Geometry check sheet. Reference: the model listing, model coordinates, mm. Give positions to 0.01 mm unless a question says otherwise; leave off trailing zeros. Loops run counter-clockwise (first coordinate to the right, second up) from the corner with the lowest first, then second, coordinate; pieces in that order, holes last. Notation, with made-up numbers: (10, 80) -> (15, 80) arc R16 ccw to (15, 94) -> close; hole circle Ø7 at (-15.75, 33.25). An arc over 180 degrees is marked (long way). One line per item, written item: value. Start each with the question number.
(1) Sectioned sample at B-B, the plane z = -124. Record the cut outline in (x, y), then the cut area to 3 significant figures.
(2) Draft check along Z on faces 1 (the face through (15.83, 103.48, -178.32)), 2 (the face through (15.83, 11.61, -171.28)), 3 (the face through (15.8, 89.7, -146.8)), 4 (the face through (15.83, 34.47, -118.71)). Enter one of: pulls with the +Z half, pulls with the -Z half, needs draft (parallel to the pull), parting line crosses it, or undercut.
(3) Sectioned sample at A-A, the plane y = 65.5. Record the cut outline in (x, z), then the cut area to 3 significant figures.
(4) Scan lines: line 1 along Z through (x, y) = (14.5, 36.5); line 2 along Z through (x, y) = (16.25, 58.5); line 3 along Y through (x, z) = (15, -130). Record each from-to range of solid material in increasing order. Write a range as from..to.
(5) Sectioned sample at C-C, the plane z = -134.5. Record the cut outline in (x, y).
(6) Sectioned sample at D-D, the plane x = 14.5. State how many separate pieces and enclosed holes the cut face has, then the cut area to 3 significant figures.
Autodesk Inventor part; units mm, degrees
ref_plane "Work Plane1" through (12.7, 0, 0) normal (1, 0, 0) x (0, 0, -1)
ref_plane "YZ Plane" through (0, 0, 0) normal (1, 0, 0) x (0, 1, 0)
ref_plane "XZ Plane" through (0, 0, 0) normal (0, 1, 0) x (-1, 0, 0)
sketch "Sketch1" plane through (0, 0, 0) normal (1, 0, 0) x (0, 1, 0)
  line L0 (111.125, 190.5) -> (68.3957, 190.5)
  line L1 (20.2274, 160.5064) -> (-11.1661, 102.5705)
  arc A0 (-11.1661, 102.5705) -> (-11.1661, 90.4695) centre (0, 96.52) ccw
  line L2 (-11.1661, 90.4695) -> (7.6076, 55.8231)
  arc A1 (-11.1661, 6.0505) -> (-11.1661, -6.0505) centre (0, 0) ccw
  line L3 (-11.1661, -6.0505) -> (7.6076, -40.6969)
  arc A2 (-11.1661, -90.4695) -> (-11.3095, -102.2979) centre (0, -96.52) ccw
  line L4 (-11.3095, -102.2979) -> (18.6694, -160.9782)
  line L5 (67.5494, -190.5) -> (111.125, -190.5)
  line L6 (111.125, -190.5) -> (111.125, 190.5)
  arc A3 (20.2274, 160.5064) -> (68.3957, 190.5) centre (42.5128, 178.392) ccw
  arc A4 (67.5494, -190.5) -> (18.6694, -160.9782) centre (42.5128, -176.727) ccw
  circle A5 centre (42.5128, 178.392) radius 4.7625 construction
  circle A6 centre (34.925, -92.075) radius 7.9375
  circle A7 centre (73.5908, -125.0234) radius 6.35 construction
  circle A8 centre (42.5128, -176.727) radius 4.7625 construction
  line L7 (111.125, 0) -> (0, 0) construction
  circle A9 centre (0, 96.52) radius 2.4892 construction
  circle A10 centre (0, 0) radius 2.4892 construction
  circle A11 centre (0, -96.52) radius 2.4892 construction
  line L8 (-11.1661, 6.0505) -> (7.6076, 40.6969)
  arc A12 (7.6076, 40.6969) -> (7.6076, 55.8231) centre (-6.35, 48.26) ccw
  line L9 (-11.1661, -90.4695) -> (7.6076, -55.8231)
  arc A13 (7.6076, -55.8231) -> (7.6076, -40.6969) centre (-6.35, -48.26) ccw
  line L10 (-6.35, -48.26) -> (-6.35, 48.26) construction
  line L11 (-6.35, 0) -> (0, 0) construction
  circle A14 centre (0, 96.52) radius 3.175
  circle A15 centre (0, 0) radius 3.175
  circle A16 centre (0, -96.52) radius 3.175
  circle A17 centre (46.0375, 122.682) radius 3.5687 construction
  circle A18 centre (20.6375, 122.682) radius 3.5687 construction
  circle A19 centre (46.0375, 122.682) radius 3.175
  circle A20 centre (20.6375, 122.682) radius 3.175
  line L12 (0, 96.52) -> (-12.7, 96.52) construction
  circle A21 centre (99.3625, 57.065) radius 2.0193
  circle A22 centre (47.625, -17.78) radius 2.0193
  circle A23 centre (99.3625, 31.665) radius 2.0193
  circle A24 centre (73.9625, 57.065) radius 2.0193
  circle A25 centre (73.9625, 31.665) radius 2.0193
  circle A26 centre (47.625, -43.18) radius 2.0193
  circle A27 centre (22.225, -17.78) radius 2.0193
  circle A28 centre (22.225, -43.18) radius 2.0193
  circle A29 centre (85.725, 107.103) radius 7.9375
  line L13 (-12.7, 173.6352) -> (-12.7, -210.2893) construction
  circle A30 centre (85.725, 107.103) radius 17.78 construction
  circle A31 centre (79.375, 147.2439) radius 22.86 construction
  circle A32 centre (42.5128, 178.392) radius 25.4 construction
  line L14 (110.475, 71.035) -> (60.975, 71.035) construction
  line L15 (60.975, 71.035) -> (60.975, -72.669) construction
  line L16 (60.975, -72.669) -> (110.475, -72.669) construction
  line L17 (110.475, -72.669) -> (110.475, 71.035) construction
  line L18 (58.7375, 86.554) -> (9.2375, 86.554) construction
  line L19 (9.2375, 86.554) -> (9.2375, -57.15) construction
  line L20 (9.2375, -57.15) -> (58.7375, -57.15) construction
  line L21 (58.7375, -57.15) -> (58.7375, 86.554) construction
  line L22 (9.525, 127) -> (-15.875, 127) construction
  line L23 (-15.875, 127) -> (-15.875, -177.8) construction
  line L24 (-15.875, -177.8) -> (9.525, -177.8) construction
  line L25 (9.525, -177.8) -> (9.525, 127) construction
  circle A33 centre (34.925, -92.075) radius 17.78 construction
  circle A34 centre (73.5908, -125.0234) radius 28.575 construction
  circle A35 centre (42.5128, -176.727) radius 31.75 construction
  circle A36 centre (102.0089, 180.2336) radius 2.413
  circle A37 centre (89.3089, 182.1987) radius 2.413
  circle A38 centre (102.0089, -180.2336) radius 2.413
  circle A39 centre (89.3089, -182.1987) radius 2.413
  circle A40 centre (79.375, 147.2439) radius 14.2875
  circle A41 centre (66.675, 254) radius 60.325 construction
  circle A42 centre (66.675, -254) radius 60.325 construction
  circle A43 centre (73.5908, -125.0234) radius 14.2875
  circle A44 centre (80.899, -155.6385) radius 47.527 construction
  circle A45 centre (100.0125, -85.369) radius 3.175
  circle A46 centre (74.6125, -85.369) radius 3.175
  circle A47 centre (100.0125, -85.369) radius 6.35 construction
  circle A48 centre (74.6125, -85.369) radius 6.35 construction
  circle A49 centre (46.0375, 122.682) radius 6.35 construction
  circle A50 centre (20.6375, 122.682) radius 6.35 construction
  circle A51 centre (34.6075, -121.8815) radius 3.175
  circle A52 centre (17.4625, -121.8815) radius 3.175
  circle A53 centre (34.6075, -121.8815) radius 6.35 construction
  circle A54 centre (17.4625, -121.8815) radius 6.35 construction
  circle A55 centre (101.6, 78.9725) radius 3.175
  circle A56 centre (101.6, 78.9725) radius 6.35 construction
  line L26 (92.075, 107.103) -> (79.375, 107.103) construction
  line L27 (79.375, 107.103) -> (79.375, 71.035) construction
  line L28 (79.375, 71.035) -> (92.075, 71.035) construction
  line L29 (92.075, 71.035) -> (92.075, 107.103) construction
  line L30 (85.725, 107.103) -> (85.725, 71.035) construction
  circle A57 centre (69.85, 78.9725) radius 3.175
  circle A58 centre (69.85, 78.9725) radius 6.35 construction
  circle A59 centre (59.143, -124.7108) radius 14.2875
  circle A60 centre (59.143, -124.7108) radius 22.86 construction
  dimension "d2" = 15.875
  dimension "d3" = 6.35
  dimension "d4" = 96.52
  dimension "d8" = 6.35
  dimension "d9" = 381
  dimension "d11" = 28.575
  dimension "d12" = 12.7
  dimension "d135" = 4.0386
  dimension "d136" = 4.0386
  dimension "d139" = 25.4
  dimension "d142" = 25.4
  dimension "d147" = 25.4
  dimension "d150" = 25.4
  dimension "d155" = 12.7
  dimension "d156" = 48.895
  dimension "d225" = 15.875
  dimension "d226" = 25.4
  dimension "d227" = 50.038
  dimension "d229" = 123.825
  dimension "d230" = 35.56
  dimension "d231" = 45.72
  dimension "d232" = 50.8
  dimension "d233" = 49.5
  dimension "d234" = 143.704
  dimension "d235" = 13.97
  dimension "d236" = 11.1125
  dimension "d237" = 143.704
  dimension "d238" = 49.5
  dimension "d239" = 11.1125
  dimension "d240" = 13.97
  dimension "d242" = 25.4
  dimension "d243" = 304.8
  dimension "d245" = 9.525
  dimension "d246" = 35.56
  dimension "d247" = 57.15
  dimension "d248" = 63.5
  dimension "d249" = 28.575
  dimension "d250" = 31.75
  dimension "d251" = 4.826
  dimension "d252" = 4.826
  dimension "d253" = 4.826
  dimension "d254" = 4.826
  dimension "d256" = 9.1161
  dimension "d257" = 12.7
  dimension "d258" = 1.9652
  dimension "d259" = 10.2664
  dimension "d260" = 12.7
  dimension "d261" = 1.9652
  dimension "d262" = 9.1161
  dimension "d263" = 10.2664
  dimension "d264" = 120.65
  dimension "d265" = 120.65
  dimension "d266" = 44.45
  dimension "d267" = 63.5
  dimension "d268" = 63.5
  dimension "d269" = 28.575
  dimension "d270" = 98.3615
  dimension "d271" = 14.224
  dimension "d272" = 95.054
  dimension "d273" = 6.35
  dimension "d274" = 6.35
  dimension "d275" = 25.4
  dimension "d276" = 11.1125
  dimension "d277" = 12.7
ref_plane "Work Plane1" through (12.7, 0, 0) normal (1, 0, 0) x (0, 0, -1)
sketch "Sketch13" plane through (12.7, 0, 0) normal (1, 0, 0) x (0, 0, -1)
  circle A0 centre (180.2336, 102.0089) radius 2.413
  circle A1 centre (182.1987, 89.3089) radius 2.413
  circle A2 centre (176.727, 42.5128) radius 4.7625 construction
  line L0 (177.8, 9.525) -> (-127, 9.525) construction
  line L1 (177.8, -15.875) -> (177.8, 9.525) construction
  circle A3 centre (121.8815, 34.6075) radius 3.175
  circle A4 centre (121.8815, 17.4625) radius 3.175
  line L2 (190.5, 111.125) -> (-190.5, 111.125)
  line L3 (190.5, 72.4418) -> (190.5, 111.125)
  circle A5 centre (124.7108, 59.143) radius 15.875
  circle A6 centre (180.2336, 102.0089) radius 5.588
  circle A7 centre (182.1987, 89.3089) radius 5.588
  circle A8 centre (176.727, 42.5128) radius 7.9375
  circle A9 centre (121.8815, 34.6075) radius 6.35
  circle A10 centre (121.8815, 17.4625) radius 6.35
  circle A11 centre (125.0234, 73.5908) radius 28.575 construction
  circle A12 centre (92.075, 34.925) radius 22.225 construction
  circle A13 centre (176.727, 42.5128) radius 31.75 construction
  line L4 (116.9572, 72.9957) -> (177.5043, 106.8851)
  line L5 (180.2336, 107.5969) -> (190.5, 107.5969)
  line L6 (168.8197, 11.1125) -> (113.2813, 11.1125)
  line L7 (108.9055, 57.6571) -> (113.2813, 11.1125)
  line L8 (173.3099, 12.9724) -> (188.6401, 28.3026)
  line L9 (190.5, 72.4418) -> (190.5, 32.7928)
  arc A14 (168.8197, 11.1125) -> (173.3099, 12.9724) centre (168.8197, 17.4625) ccw
  arc A15 (188.6401, 28.3026) -> (190.5, 32.7928) centre (184.15, 32.7928) ccw
  circle A16 centre (124.7108, 59.143) radius 14.2875
  point P0 (0, 0)
  point P1 (190.5, 30.1625)
  point P2 (171.45, 11.1125)
  point P3 (121.8815, 11.1125)
  dimension "d299" = 3.175
  dimension "d300" = 3.175
  dimension "d303" = 15.875
  dimension "d304" = 12.7
  dimension "d305" = 12.7
  dimension "d307" = 19.05
  dimension "d308" = 19.05
  dimension "d309" = 6.35
  dimension "d310" = 6.35
  dimension "d313" = 31.75
extrude "Extrusion14" add sketch "Sketch13" along normal blind 6.35 contours A10 | L9 A15 L8 A14 L6 L7 A5 L4 A6 L5 L3 | A6 | A5 | A7 | A9
properties part number "OuterDriveRail" material "Aluminum 6061"
Calculated:
1. outline: (12.7, 11.11) -> (19.05, 11.11) -> (19.05, 15.1) -> (12.7, 15.1) -> close; (12.7, 19.83) -> (19.05, 19.83) -> (19.05, 32.24) -> (12.7, 32.24) -> close; (12.7, 36.97) -> (19.05, 36.97) -> (19.05, 44.87) -> (12.7, 44.87) -> close; (12.7, 73.41) -> (19.05, 73.41) -> (19.05, 76.94) -> (12.7, 76.94) -> close
1. area: 177 mm2
2. face 1: undercut
2. face 2: pulls with the -Z half
2. face 3: pulls with the +Z half
2. face 4: undercut
3. outline: (12.7, -190.5) -> (19.05, -190.5) -> (19.05, -137.51) -> (12.7, -137.51) -> close; (12.7, -111.92) -> (19.05, -111.92) -> (19.05, -110.16) -> (12.7, -110.16) -> close
3. area: 348 mm2
4. line 1: z = -190.5..-181.91, -171.55..-124.43, -119.33..-110.89
4. line 2: z = -190.5..-138.98, -110.44..-108.85
4. line 3: y = 11.11..45.87, 72.42..80.3
5. outline: (12.7, 11.11) -> (19.05, 11.11) -> (19.05, 48.74) -> (12.7, 48.74) -> close; (12.7, 69.55) -> (19.05, 69.55) -> (19.05, 82.81) -> (12.7, 82.81) -> close
6. separate pieces: 1
6. enclosed holes: 6
6. area: 5,270 mm2
